Geometry check sheet. Reference: the model listing, model coordinates, mm. Face numbers are marked on the shaded views. Give positions to 0.01 mm unless a question says otherwise; leave off trailing zeros. Loops run counter-clockwise (first coordinate to the right, second up) from the corner with the lowest first, then second, coordinate; pieces in that order, holes last.
1. Cross-section at B-B, the plane z = -6.5. Record the cut outline in (x, y), plus the area to 3 significant figures.
2. Go/stop test with flat-tipped pins: pin 1 Ø8 at (y, z) = (40.5, 2) entering from +X; pin 2 Ø7.5 at (y, z) = (-6.5, -2.5) entering from -X; pin 3 Ø18 at (x, y) = (2, -15) entering from -Z; pin 4 Ø4.5 at (x, y) = (22.225, 0) entering from -Z. Record where each tip stops, or that it passes through.
3. Material ranges on L1, parallel to Y at x = 0, z = 8.9 (1 decimal); L2, parallel to Y at x = -152.4, z = 0.55 (3 decimals); L3, parallel to Z at x = -104, y = 31 (1 decimal), recorded low to high.
4. Cross-section at C-C, the plane x = -73. Record the cut outline in (y, z) (1 decimal).
5. Release check for a two-part mould opening along X. For the marked faces 1 and 2 record: +X half, -X half, draft (parallel to the pull), parting line (faces both ways), or undercut.
from build123d import *

# Parameters (mm, degrees)
SKETCH1_R               = 31.75
SKETCH1_R_2             = 12.7
SKETCH1_R_3             = 2.54
BOSS_EXTRUDE1_DEPTH     = 1.5875
SKETCH3_W               = 635
SKETCH3_H               = 144.4625
SKETCH3_R               = 29.21
BOSS_EXTRUDE2_DEPTH     = 1.5875
SKETCH4_R               = 41.275
SKETCH5_R               = 31.75
SKETCH6_R               = 30.1625
TIMER_HOLE_DEPTH        = 6.35
SKETCH7_W               = 19.05
SKETCH7_H               = 38.1
SOAK_LIGHT_DEPTH        = 25.4
SKETCH8_R               = 44.45
SKETCH9_R               = 31.75
SKETCH10_R              = 31.75
CUT_EXTRUDE1_DEPTH      = 6.35
CUT_EXTRUDE1_DEPTH_BACK = 2.5875
SKETCH11_R              = 1.651
CUT_EXTRUDE2_DEPTH      = 10.525


with BuildPart() as part:
    # Sketch1 → Boss-Extrude1 (new body)
    with BuildSketch(Plane.XY):
        Circle(SKETCH1_R)
        Circle(SKETCH1_R_2, mode=Mode.SUBTRACT)
        with Locations((-22.225, 0)):
            Circle(SKETCH1_R_3, mode=Mode.SUBTRACT)
        with Locations((22.225, 0)):
            Circle(SKETCH1_R_3, mode=Mode.SUBTRACT)
    extrude(amount=BOSS_EXTRUDE1_DEPTH)



with BuildPart() as body_2:
    # Sketch3 → Boss-Extrude2 (new body)
    with BuildSketch(Plane.XY.offset(7.9375)):
        with Locations((-187.325, 5.55625)):
            Rectangle(SKETCH3_W, SKETCH3_H)
        Circle(SKETCH3_R, mode=Mode.SUBTRACT)
    extrude(amount=BOSS_EXTRUDE2_DEPTH)


with BuildPart() as part_1:
    add(part.part)

    add(body_2.part)  # Loft1 merges body 2
    # Sketch4 → Loft1 section 0
    with BuildSketch(Plane(origin=(0, 0, 7.9375), x_dir=(-1, 0, 0), z_dir=(0, 0, -1))):
        Circle(SKETCH4_R)
    # Sketch5 → Loft1 section 1
    with BuildSketch(Plane(origin=(0, 0, 1.5875), x_dir=(-1, 0, 0), z_dir=(0, 0, -1))):
        Circle(SKETCH5_R)
    loft()

    # Sketch6 → Timer hole (cut)
    with BuildSketch(Plane(origin=(0, 0, 7.9375), x_dir=(-1, 0, 0), z_dir=(0, 0, -1))):
        Circle(SKETCH6_R)
    extrude(amount=TIMER_HOLE_DEPTH, mode=Mode.SUBTRACT)

    # Sketch7 → Soak light (add)
    with BuildSketch(Plane(origin=(0, 0, 7.9375), x_dir=(-1, 0, 0), z_dir=(0, 0, -1))):
        with Locations((-104.775, 0)):
            Rectangle(SKETCH7_W, SKETCH7_H)
    extrude(amount=SOAK_LIGHT_DEPTH)

    # Sketch8 → spare mount section 0
    with BuildSketch(Plane(origin=(0, 0, 7.9375), x_dir=(-1, 0, 0), z_dir=(0, 0, -1))):
        with Locations((152.4, 17.145)):
            Circle(SKETCH8_R)
    # Sketch9 → spare mount section 1
    with BuildSketch(Plane(origin=(0, 0, 0), x_dir=(-1, 0, 0), z_dir=(0, 0, -1))):
        with Locations((152.4, 17.145)):
            Circle(SKETCH9_R)
    loft()

    # Sketch10 → Cut-Extrude1 (cut, two sides)
    with BuildSketch(Plane(origin=(0, 0, 7.9375), x_dir=(-1, 0, 0), z_dir=(0, 0, -1))) as cut_extrude1_sk:
        with Locations((152.4, 17.145)):
            Circle(SKETCH10_R)
    extrude(amount=CUT_EXTRUDE1_DEPTH, mode=Mode.SUBTRACT)
    extrude(cut_extrude1_sk.sketch, amount=-CUT_EXTRUDE1_DEPTH_BACK, mode=Mode.SUBTRACT)

    # Sketch11 → Cut-Extrude2 (cut, through all)
    with BuildSketch(Plane(origin=(0, 0, 0), x_dir=(-1, 0, 0), z_dir=(0, 0, -1))):
        with Locations((152.4, 26.416)):
            Circle(SKETCH11_R)
        with Locations((152.4, 38.735)):
            Circle(SKETCH11_R)
    extrude(amount=-CUT_EXTRUDE2_DEPTH, mode=Mode.SUBTRACT)


solid = part_1.part
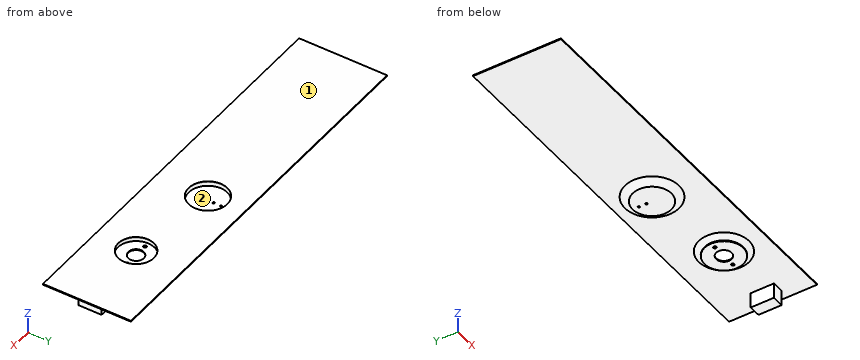
Result:
1. outline: (95.25, -19.05) - (114.3, -19.05) - (114.3, 19.05) - (95.25, 19.05) - close
1. area: 726 mm2
2. pin 1: stops at x = -117.83
2. pin 2: stops at x = -177.2
2. pin 3: stops at z = 0
2. pin 4: passes through
3. L1: y = -66.7 to -29.2, 29.2 to 77.8
3. L2: y = -15.485 to 24.765, 28.067 to 37.084, 40.386 to 49.775
3. L3: z = 7.9 to 9.5
4. outline: (-66.7, 7.9) - (77.8, 7.9) - (77.8, 9.5) - (-66.7, 9.5) - close
5. face 1: draft
5. face 2: undercut
